```python
from build123d import *

# Parameters (mm, degrees)
EXTRUDE_1_DEPTH     = 4
SKETCH_2_R          = 1.5
CUT_EXTRUDE_1_DEPTH = 4
SKETCH_3_R          = 1.5
CUT_EXTRUDE_2_DEPTH = 4


with BuildPart() as part:
    # 草图1 → 凸台-拉伸1 (new body)
    with BuildSketch(Plane(origin=(0, 0, 0), x_dir=(1, 0, 0), z_dir=(0, 1, 0))):
        with BuildLine():
            Line((-0.120614758, 100.331386325), (-9.879385242, 127.143387869))
            ThreePointArc((-9.879385242, 127.143387869), (-9.969615506, 127.480131801), (-10, 127.827428156))
            Line((-10, 127.827428156), (-10, 152.949548389))
            ThreePointArc((-10, 152.949548389), (-9.414213562, 154.363761951), (-8, 154.949548389))
            Line((-8, 154.949548389), (68, 154.949548389))
            ThreePointArc((68, 154.949548389), (69.414213562, 154.363761951), (70, 152.949548389))
            Line((70, 152.949548389), (70, 127.827428156))
            ThreePointArc((70, 127.827428156), (69.969615506, 127.480131801), (69.879385242, 127.143387869))
            Line((69.879385242, 127.143387869), (60.120614758, 100.331386325))
            ThreePointArc((60.120614758, 100.331386325), (60.030384494, 99.994642394), (60, 99.647346039))
            Line((60, 99.647346039), (60, 2))
            ThreePointArc((60, 2), (59.414213562, 0.585786438), (58, 0))
            Line((58, 0), (2, 0))
            ThreePointArc((2, 0), (0.585786438, 0.585786438), (0, 2))
            Line((0, 2), (0, 99.647346039))
            ThreePointArc((0, 99.647346039), (-0.030384494, 99.994642394), (-0.120614758, 100.331386325))
        make_face()
    extrude(amount=EXTRUDE_1_DEPTH)

    # 草图2 → 切除-拉伸1 (cut)
    with BuildSketch(Plane(origin=(0, 4, 0), x_dir=(1, 0, 0), z_dir=(0, 1, 0))):
        with Locations(Location((10, 25, 0), (0, 0, 270))):
            Circle(SKETCH_2_R)
        with Locations(Location((34, 25, 0), (0, 0, 270))):
            Circle(SKETCH_2_R)
        with Locations(Location((34, 55, 0), (0, 0, 270))):
            Circle(SKETCH_2_R)
        with Locations(Location((10, 55, 0), (0, 0, 270))):
            Circle(SKETCH_2_R)
    extrude(amount=-CUT_EXTRUDE_1_DEPTH, mode=Mode.SUBTRACT)

    # 草图3 → 切除-拉伸2 (cut)
    with BuildSketch(Plane(origin=(0, 4, 0), x_dir=(1, 0, 0), z_dir=(0, 1, 0))):
        with Locations(Location((2, 147.449548389, 0), (0, 0, 270))):
            Circle(SKETCH_3_R)
        with Locations(Location((15, 147.449548389, 0), (0, 0, 270))):
            Circle(SKETCH_3_R)
        with Locations(Location((45, 147.449548389, 0), (0, 0, 90))):
            Circle(SKETCH_3_R)
        with Locations(Location((58, 147.449548389, 0), (0, 0, 90))):
            Circle(SKETCH_3_R)
        with Locations(Location((30, 147.449548389, 0), (0, 0, 270))):
            Circle(SKETCH_3_R)
    extrude(amount=-CUT_EXTRUDE_2_DEPTH, mode=Mode.SUBTRACT)


solid = part.part
```
Here's how the part is built. I have some questions about the finished solid (model axes, mm). A direction names the side the tool comes from. Give positions to 0.01 mm unless a question says otherwise; leave off trailing zeros. Write each loop counter-clockwise with the first axis right and the second up, starting at its lowest first coordinate (ties: lowest second). Pieces come first, ordered by that corner, then holes.
(1) On a 3-axis mill with a long thin cutter (end or side, diameter ignored), from which of +Z, -Z, +X, -X, +Y, -Y can I reach the whole of each face in a straight line? I mean faces 1 (the face through (0, 2, -50)), 2 (the face through (32.67, 2.03, -54.31)). Say none if no direction works.
Output values:
face 1: +Z, -X, +Y, -Y
face 2: +Y, -Y
(2) Imagine slicing it at D-D, the plane y = 1.25. Count the separate pieces of the cut face and the enclosed holes in it, and give its area (3 significant figures).
Output values:
separate pieces: 1
enclosed holes: 9
area: 10,100 mm2
(3) If I drill on L1, parallel to X at y = 1.7, z = -25; L2, parallel to Z at x = 11, y = 1.8; L3, parallel to Z at x = 45.5, y = 0.8, over which ranges is the centre line in solid material (lowest first)?
Output values:
L1: x = 0 to 8.5, 11.5 to 32.5, 35.5 to 60
L2: z = -154.95 to -56.12, -53.88 to -26.12, -23.88 to 0
L3: z = -154.95 to -148.86, -146.04 to 0
(4) Imagine slicing it at A-A, the plane z = -25. Write out the boundary of the cut face in (x, y), and give its area (3 significant figures).
Output values:
outline: (0, 0) - (8.5, 0) - (8.5, 4) - (0, 4) - close; (11.5, 0) - (32.5, 0) - (32.5, 4) - (11.5, 4) - close; (35.5, 0) - (60, 0) - (60, 4) - (35.5, 4) - close
area: 216 mm2
(5) Imagine slicing it at C-C, the plane x = 45. Write out the boundary of the cut face in (y, z), and give its area (3 significant figures).
Output values:
outline: (0, -154.95) - (4, -154.95) - (4, -148.95) - (0, -148.95) - close; (0, -145.95) - (4, -145.95) - (4, 0) - (0, 0) - close
area: 608 mm2
(6) Will this pin go through, and if not, where does the flat tip stop? pin 1 (2 mm diameter, centred on y = 2, z = -72, fed in from +X).
Output values:
pin 1: stops at x = 60
(7) Imagine slicing it at B-B, the plane x = 10. Write out the boundary of the cut face in (y, z), and give its area (3 significant figures).
Output values:
outline: (0, -154.95) - (4, -154.95) - (4, -56.5) - (0, -56.5) - close; (0, -53.5) - (4, -53.5) - (4, -26.5) - (0, -26.5) - close; (0, -23.5) - (4, -23.5) - (4, 0) - (0, 0) - close
area: 596 mm2
(8) Thinking about a two-plate mould opening in Z: for faces 3 (the face through (60, 2, -52)), 4 (the face through (65.07, 1.97, -113.93)), 5 (the face through (14.43, 2.03, -146.06)), 6 (the face through (10.45, 2.03, -53.57)), which applies, pulls with the +Z half, pulls with the -Z half, needs draft (parallel to the pull), parting line crosses it, or undercut?
Output values:
face 3: needs draft
face 4: pulls with the +Z half
face 5: undercut
face 6: undercut
